Verification items for the finished model (mm, model axes). A direction names the side the tool comes from. Coordinates: 2 decimals unless noted, no trailing zeros. Loops run counter-clockwise (first coordinate to the right, second up) from the corner with the lowest first, then second, coordinate; pieces in that order, holes last. Notation, with made-up numbers: (-10.75, 53.25) - (44.25, 53.25) arc R15 ccw to (44.25, 80.25) - close; hole circle Ø2 at (1, 23.25). An arc over 180 degrees is marked (long way). One line per item, written item: value. Start each with the question number.
(1) Set-up check for faces 4 (the face through (5, 6, -5)), 5 (the face through (0, -1, 6.25)), 6 (the face through (-10, 0, 2)): record each of +Z, -Z, +X, -X, +Y, -Y from which the full face is reachable in a straight line by a thin tool's end or side.
(2) Thickness scan on probe 1 along Z at (x, y) = (0, -9.5); probe 2 along Z at (x, y) = (0.25, -0.5); probe 3 along Y at (x, z) = (3.25, 4.25). Record the ranges inside material, lowest first. Write a range as [from, to].
(3) Section check B-B (z = 0.5). Record the boundary of the cut face in (x, y), plus the area to 3 significant figures.
(4) Section check A-A (x = 0). Record the boundary of the cut face in (y, z).
(5) Draft check along Z on faces 1 (the face through (5.387, -0.902, -3.169)), 2 (the face through (10.4, 3.04, -3.27)), 3 (the face through (2, -10, -2)). Enter one of: +Z half, -Z half, draft (parallel to the pull), parting line (faces both ways), or undercut.
(6) Section check C-C (y = 1.5). Record the boundary of the cut face in (x, z), plus the area to 3 significant figures.
(7) Gauge pin test, flat ends, axial feed: P1, Ø8, axis at y = 2, z = 4.5, coming from the -X side; P2, Ø5, axis at y = -6.5, z = 7.5, coming from the -X side; P3, Ø6.5, axis at x = 0, z = 0, coming from the +Y side; P4, Ø11, axis at x = -2, z = -1, coming from the -Y side. Record the tip position at first contact, or that the pin passes through.
(8) Section check D-D (x = -4.5). Record the boundary of the cut face in (y, z), plus the area to 3 significant figures.
Autodesk Inventor part; units mm, degrees
ref_plane "YZ Plane" through (0, 0, 0) normal (1, 0, 0) x (0, 1, 0)
ref_plane "XZ Plane" through (0, 0, 0) normal (0, 1, 0) x (-1, 0, 0)
ref_plane "XY Plane" through (0, 0, 0) normal (0, 0, 1) x (1, 0, 0)
sketch "Sketch2" plane through (0, 0, 0) normal (0, 0, 1) x (1, 0, 0)
  line L0 (0, 0) -> (10.9, 0)
  line L1 (10.9, 0) -> (10.9, 6)
  line L2 (10.9, 6) -> (0, 6)
  line L3 (0, 6) -> (0, 0)
  line L4 (0, 0) -> (9.8, 0)
  line L5 (9.8, 0) -> (9.8, -10)
  line L6 (9.8, -10) -> (0, -10)
  line L7 (0, -10) -> (0, 0)
  dimension "d1" = 10.9
  dimension "d2" = 6
  dimension "d3" = 9.8
  dimension "d4" = 10
revolve "Revolution1" add sketch "Sketch2" angle 360 about axis through (0, 6, 0) along (0, -1, 0)
sketch "Sketch5" plane through (0, 6, 0) normal (0, 1, 0) x (1, 0, 0)
  line L0 (3.6084, 6.25) -> (7.2169, 0)
  line L1 (7.2169, 0) -> (3.6084, -6.25)
  line L2 (3.6084, -6.25) -> (-3.6084, -6.25)
  line L3 (-3.6084, -6.25) -> (-7.2169, 0)
  line L4 (-7.2169, 0) -> (-3.6084, 6.25)
  line L5 (-3.6084, 6.25) -> (3.6084, 6.25)
  point P0 (0, 0)
  point P1 (0, 0)
  dimension "d16" = 12.5
extrude "Extrusion2" cut sketch "Sketch5" against normal blind 14
sketch "Sketch6" plane through (0, -10, 0) normal (0, -1, 0) x (1, 0, 0)
  circle A0 centre (0, 0) radius 2.5
  point P0 (0, 0)
  dimension "d19" = 5
extrude "Extrusion3" cut sketch "Sketch6" against normal through all
properties part number "WHEEL_ADAPTER"
Responses:
1. face 4: +Z, -Z, +X, -X, +Y
1. face 5: +Y
1. face 6: -Y
2. probe 1: z = [-9.8, -2.5], [2.5, 9.8]
2. probe 2: z = [-9.8, -6.25], [6.25, 9.8]
2. probe 3: y = [-10, -8]
3. outline: (-10.89, 0) - (-9.79, 0) - (-9.79, -10) - (-2.45, -10) - (-2.45, -8) - (-6.93, -8) - (-6.93, 6) - (-10.89, 6) - close; (2.45, -10) - (9.79, -10) - (9.79, 0) - (10.89, 0) - (10.89, 6) - (6.93, 6) - (6.93, -8) - (2.45, -8) - close
3. area: 123 mm²
4. outline: (-10, -9.8) - (0, -9.8) - (0, -10.9) - (6, -10.9) - (6, -6.25) - (-8, -6.25) - (-8, -2.5) - (-10, -2.5) - close; (-10, 2.5) - (-8, 2.5) - (-8, 6.25) - (6, 6.25) - (6, 10.9) - (0, 10.9) - (0, 9.8) - (-10, 9.8) - close
5. face 1: undercut
5. face 2: parting line
5. face 3: draft
6. outline: circle Ø21.8 at (0, 0); hole (-7.22, 0) - (-3.61, -6.25) - (3.61, -6.25) - (7.22, 0) - (3.61, 6.25) - (-3.61, 6.25) - close
6. area: 238 mm²
7. P1: stops at x = -10.89
7. P2: stops at x = -8.43
7. P3: stops at y = -8
7. P4: stops at y = -10
8. outline: (-10, -8.71) - (0, -8.71) - (0, -9.93) - (6, -9.93) - (6, -4.71) - (-8, -4.71) - (-8, 4.71) - (6, 4.71) - (6, 9.93) - (0, 9.93) - (0, 8.71) - (-10, 8.71) - close
8. area: 161 mm²
